Design review of the part built by this model. Coordinates are the model's own, in mm. Face numbers are marked on the shaded views. Give positions to 0.01 mm unless a question says otherwise; leave off trailing zeros. Order: outer loops, then holes, each group sorted by start corner. A loop starts at its lowest first (then second) coordinate and runs counter-clockwise, first axis right, second up. Notation, with made-up numbers: (14, -24.5) -> (36, -24.5) arc R27 ccw to (36, 13.5) -> close; hole circle Ø6 at (74, 5). An arc over 180 degrees is marked (long way). Answer in a Markdown table with one row per item. Add a question column.
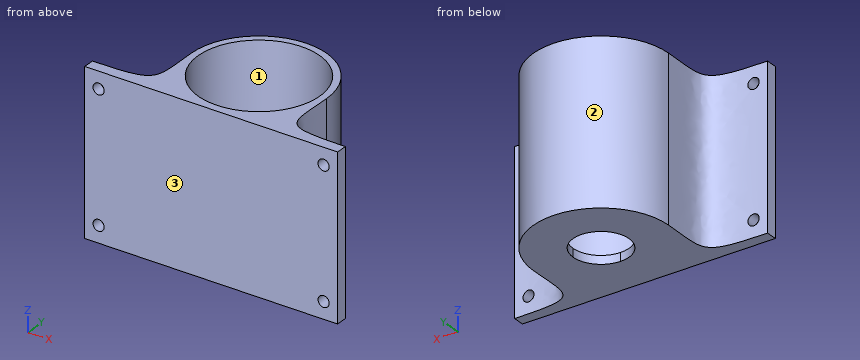
```python
from build123d import *

# Parameters (mm, degrees)
SKETCH1_R           = 24.241475666
SKETCH1_R_2         = 21.76
BOSS_EXTRUDE1_DEPTH = 58
SKETCH1_4_R         = 21.76
BOSS_EXTRUDE2_DEPTH = 3
SKETCH2_R           = 2
CUT_EXTRUDE2_DEPTH  = 30
SKETCH2_3_R         = 2.006014876
CUT_EXTRUDE3_DEPTH  = 30


with BuildPart() as part:
    # Sketch1 → Boss-Extrude1 (new body)
    # profile 1 of 2: a face of its own
    with BuildSketch(Plane.XY):
        Circle(SKETCH1_R)
        with Locations(Location((0, 0, 0), (0, 0, 180))):
            Circle(SKETCH1_R_2, mode=Mode.SUBTRACT)
    # profile 2 of 2: a face of its own
    with BuildSketch(Plane.XY):
        with BuildLine():
            Line((-45.421940828, -20.666245921), (-45.421940828, -24.666245921))
            Line((-45.421940828, -24.666245921), (45.421940828, -24.666245921))
            Line((45.421940828, -24.666245921), (45.421940828, -20.666245921))
            add(Edge.make_bspline(
                [(45.421940828, -20.666245921), (21.532203305, -20.666245921), (24.241475666, -19.078845964), (24.241475666, 0)],
                knots=[0, 0, 0, 0, 1, 1, 1, 1], degree=3))
            ThreePointArc((24.241475666, 0), (0, -24.241475666), (-24.241475666, 0))
            add(Edge.make_bspline(
                [(-45.421940828, -20.666245921), (-21.532203305, -20.666245921), (-24.241475666, -19.078845964), (-24.241475666, 0)],
                knots=[0, 0, 0, 0, 1, 1, 1, 1], degree=3))
        make_face()
    extrude(amount=BOSS_EXTRUDE1_DEPTH)

    # Sketch1_4 → Boss-Extrude2 (add)
    with BuildSketch(Plane.XY):
        with Locations(Location((0, 0, 0), (0, 0, 180))):
            Circle(SKETCH1_4_R)
        with BuildLine():
            ThreePointArc((0, -10), (-7.071067812, 7.071067812), (10, 0))
            ThreePointArc((10, 0), (7.071067812, -7.071067812), (0, -10))
        make_face(mode=Mode.SUBTRACT)
    extrude(amount=BOSS_EXTRUDE2_DEPTH)

    # Sketch2 → Cut-Extrude2 (cut)
    with BuildSketch(Plane(origin=(0, 0, 0), x_dir=(1, 0, 0), z_dir=(0, 1, 0))):
        with Locations(Location((-40.421940828, -6, 0), (0, 0, 270))):
            Circle(SKETCH2_R)
        with Locations(Location((40.421940828, -6, 0), (0, 0, 270))):
            Circle(SKETCH2_R)
    extrude(amount=-CUT_EXTRUDE2_DEPTH, mode=Mode.SUBTRACT)

    # Sketch2_3 → Cut-Extrude3 (cut)
    with BuildSketch(Plane(origin=(0, 0, 0), x_dir=(1, 0, 0), z_dir=(0, 1, 0))):
        with Locations(Location((-40.421940828, -52, 0), (0, 0, 270))):
            Circle(SKETCH2_3_R)
        with Locations(Location((40.421940828, -52, 0), (0, 0, 270))):
            Circle(SKETCH2_3_R)
    extrude(amount=-CUT_EXTRUDE3_DEPTH, mode=Mode.SUBTRACT)


solid = part.part
```
1) Add section C-C, the plane z = 6. Give the number of separate pieces and of enclosed holes in the cut face, and give its area (3 significant figures).
2) Clearance check with flat-ended pins moving along their axes: P1, Ø3, axis at x = 40.42, z = 52, coming from the +Y side; P2, Ø3, axis at y = 14.5, z = 10.5, coming from the -X side. State where each tip first meets the part, or that it passes through.
3) Add section A-A, the plane x = -7. Write out the cut boundary in (y, z).
4) Add section B-B, the plane y = 4. Write out the cut boundary in (x, z).
5) For L1, parallel to X at y = -22, z = 6; L2, parallel to Y at x = 0, z = 1; L3, parallel to Z at x = -8, y = -8, list the stretches that pass through material, from the lowest coordinate up.
6) Add section D-D, the plane x = -19. Write out the cut boundary in (y, z).
7) Mouldability with a two-part tool opening along X and no side actions: class the marked faces 1, 2 and 3 as +X half, -X half, draft (parallel to the pull), parting line (faces both ways), or undercut.
Verdict:
| question | item | result |
|---|---|---|
| 1 | separate pieces | 3 |
| 1 | enclosed holes | 1 |
| 1 | area | 804 mm2 |
| 2 | P1 | passes through |
| 2 | P2 | stops at x = -20.46 |
| 3 | outline | (-24.67, 0) -> (-7.14, 0) -> (-7.14, 3) -> (-20.6, 3) -> (-20.6, 58) -> (-24.67, 58) -> close; (7.14, 0) -> (23.21, 0) -> (23.21, 58) -> (20.6, 58) -> (20.6, 3) -> (7.14, 3) -> close |
| 4 | outline | (-23.91, 0) -> (-9.17, 0) -> (-9.17, 3) -> (-21.39, 3) -> (-21.39, 58) -> (-23.91, 58) -> close; (9.17, 0) -> (23.91, 0) -> (23.91, 58) -> (21.39, 58) -> (21.39, 3) -> (9.17, 3) -> close |
| 5 | L1 | x = -45.42 to -42.42, -38.42 to 38.42, 42.42 to 45.42 |
| 5 | L2 | y = -24.67 to -10, 10 to 24.24 |
| 5 | L3 | z = 0 to 3 |
| 6 | outline | (-24.67, 0) -> (15.05, 0) -> (15.05, 58) -> (10.61, 58) -> (10.61, 3) -> (-10.61, 3) -> (-10.61, 58) -> (-24.67, 58) -> close |
| 7 | face 1 | undercut |
| 7 | face 2 | parting line |
| 7 | face 3 | draft |
